Design review of the part built by this model. Coordinates are the model's own, in mm. A direction names the side the tool comes from. Coordinates: 2 decimals unless noted, no trailing zeros. Loops run counter-clockwise (first coordinate to the right, second up) from the corner with the lowest first, then second, coordinate; pieces in that order, holes last. Notation, with made-up numbers: (40.5, -12) -> (71.5, -12) arc R19 ccw to (71.5, 3) -> close; hole circle Ø6 at (30.5, 65). An arc over 180 degrees is marked (long way). One line per item, written item: value. Start each with the question number.
1. Add section A-A on y = 0. Write out the cut boundary in (x, z), plus the area to 3 significant figures.
2. Add section D-D on y = 8. Write out the cut boundary in (x, z).
3. Insertion check: pin 1 (3 mm diameter, centred on x = -20.5, y = -6.5, fed in from +Z); pin 2 (2.5 mm diameter, centred on y = -5, z = 9, fed in from +X); pin 3 (3 mm diameter, centred on x = -3, y = -9, fed in from +Z); pin 4 (2.5 mm diameter, centred on y = -11, z = 4.5, fed in from -X). Each pin has a flat end and moves straight along its axis. Give the tip position at first contact, or say it passes through.
4. Add section C-C on z = 9.5. Write out the cut boundary in (x, y).
5. Draft analysis for pull direction Z (two halves, no side actions). For faces 1 (the flat face through (-13.2, 0.2, 7.8)), 2 (the flat face through (-9, 14.5, 5)), 3 (the flat face through (-14, -4, 4)), 4 (the flat face through (-14, 0, 6.1)), state which applies: pulls with the +Z half, pulls with the -Z half, needs draft (parallel to the pull), parting line crosses it, or undercut.
6. Add section B-B on x = -6.5. Write out the cut boundary in (y, z).
7. For probe 1 along Y at (x, z) = (-8, 4.25); probe 2 along Y at (x, z) = (-14, 10); probe 3 along X at (y, z) = (-11.25, 10), list the stretches that pass through material, from the lowest coordinate up.
8. Machinability: for faces 5 (the flat face through (-4, -10, 4)), 6 (the flat face through (-18, 10, 5)), 7 (the flat face through (-14, 4, 4)), 8 (the flat face through (-15.65, 0, 9)), 9 (the flat face through (-18, -11, 5)), which of the approach directions +Z, -Z, +X, -X, +Y, -Y give a long, thin tool a straight path to every point of the face, cutting with its end or side? Answer none if there is none.
Autodesk Inventor part; units mm, degrees
ref_plane "YZ Plane" through (0, 0, 0) normal (1, 0, 0) x (0, 1, 0)
ref_plane "XZ Plane" through (0, 0, 0) normal (0, 1, 0) x (-1, 0, 0)
ref_plane "XY Plane" through (0, 0, 0) normal (0, 0, 1) x (1, 0, 0)
sketch "Sketch2" plane through (0, 0, 0) normal (0, 0, 1) x (1, 0, 0)
  line L0 (-18, 14.5) -> (18, 14.5)
  line L1 (18, 14.5) -> (18, -14.5)
  line L2 (18, -14.5) -> (-18, -14.5)
  line L3 (-18, -14.5) -> (-18, 14.5)
  line L4 (-18, 14.5) -> (18, -14.5) construction
  line L5 (18, 14.5) -> (-18, -14.5) construction
  point P0 (0, 0)
  dimension "d0" = 29
  dimension "d1" = 36
extrude "Extrusion1" add sketch "Sketch2" along normal blind 11
sketch "Sketch3" plane through (0, 0, 11) normal (0, 0, 1) x (1, 0, 0)
  line L0 (-15.65, 12.15) -> (15.65, 12.15)
  line L1 (15.65, 12.15) -> (15.65, -12.15)
  line L2 (15.65, -12.15) -> (-15.65, -12.15)
  line L3 (-15.65, -12.15) -> (-15.65, 12.15)
  line L4 (-15.65, 12.15) -> (15.65, -12.15) construction
  line L5 (15.65, 12.15) -> (-15.65, -12.15) construction
  point P0 (0, 0)
  dimension "d4" = 31.3
  dimension "d5" = 24.3
extrude "Extrusion2" cut sketch "Sketch3" against normal blind 3.2
sketch "Sketch4" plane through (0, 0, 7.8) normal (0, 0, 1) x (1, 0, 0)
  line L0 (-8, 10) -> (8, 10)
  line L1 (13, 5) -> (13, -6)
  line L2 (9, -10) -> (-9, -10)
  line L3 (-13, -6) -> (-13, 5)
  line L4 (-13, 10) -> (13, -10) construction
  line L5 (13, 10) -> (-13, -10) construction
  line L6 (-13, 5) -> (-8, 10)
  line L7 (8, 10) -> (13, 5)
  arc A0 (-13, -6) -> (-9, -10) centre (-9, -6) ccw
  arc A1 (9, -10) -> (13, -6) centre (9, -6) ccw
  point P0 (0, 0)
  point P1 (-13, -4)
  point P2 (13, -4)
  dimension "d8" = 26
  dimension "d9" = 20
  dimension "d10" = 5
  dimension "d11" = 5
  dimension "d12" = 5
  dimension "d13" = 5
  dimension "d14" = 4
extrude "Extrusion3" cut sketch "Sketch4" against normal through all
sketch "Sketch6" plane through (0, 0, 0) normal (0, 1, 0) x (-1, 0, 0)
  line L0 (13, 7.8) -> (13, 0)
  line L1 (13, 6.1) -> (15.1, 6.1)
  line L2 (15.1, 6.1) -> (13, 1.1)
  line L3 (13, 1.1) -> (13, 6.1)
  line L4 (15.65, 7.8) -> (-15.65, 7.8)
  line L5 (0, 0) -> (0, 10.1915) construction
  line L6 (-13, 7.8) -> (-13, 0)
  line L7 (-13, 6.1) -> (-15.1, 6.1)
  line L8 (-15.1, 6.1) -> (-13, 1.1)
  line L9 (-13, 1.1) -> (-13, 6.1)
  line L10 (-15.65, 7.8) -> (15.65, 7.8)
  dimension "d23" = 2.1
  dimension "d24" = 5
  dimension "d25" = 1.7
extrude "Extrusion5" cut sketch "Sketch6" along normal mid plane 8
sketch "Sketch7" plane through (0, 0, 11) normal (0, 0, 1) x (1, 0, 0)
  arc A0 (21.3831, -3.7533) -> (21.3831, 3.7533) centre (20, 0) ccw
  line L0 (21.3831, 3.7533) -> (18, 5)
  line L1 (18, 5) -> (18, -5)
  line L2 (13, 5) -> (13, -6)
  line L3 (18, -5) -> (21.3831, -3.7533)
  line L4 (0, 20.7674) -> (0, -20.7674) construction
  arc A1 (-21.3831, 3.7533) -> (-21.3831, -3.7533) centre (-20, 0) ccw
  line L5 (-21.3831, 3.7533) -> (-18, 5)
  line L6 (-18, 5) -> (-18, -5)
  line L7 (-18, -5) -> (-21.3831, -3.7533)
  line L8 (18, -14.5) -> (18, 14.5) construction
  circle A2 centre (20, 0) radius 1.65
  circle A3 centre (-20, 0) radius 1.65
  line L9 (0, 0) -> (1.9739, 0) construction
  dimension "d28" = 3.3
  dimension "d29" = 4
  dimension "d30" = 40
  dimension "d31" = 10
extrude "Extrusion6" add sketch "Sketch7" against normal up to surface (11 mm away)
fillet "Fillet1" radius 2 4 edges at (18, -5, 5.5) (18, 5, 5.5) (-18, 5, 5.5) (-18, -5, 5.5)
sketch "Sketch8" plane through (0, 0, 0) normal (1, 0, 0) x (0, 1, 0)
  line L0 (45.1511, -28.2394) -> (-45.1511, -28.2394)
  line L1 (-45.1511, -28.2394) -> (-45.1511, 28.2394)
  line L2 (-45.1511, 28.2394) -> (45.1511, 28.2394)
  line L3 (45.1511, 28.2394) -> (45.1511, -28.2394)
  line L4 (45.1511, -28.2394) -> (-45.1511, 28.2394) construction
  line L5 (-45.1511, -28.2394) -> (45.1511, 28.2394) construction
  point P0 (0, 0)
extrude "Extrusion7" cut sketch "Sketch8" along normal through all
equation "\"d11\" = d10"
equation "\"d12\" = d10"
equation "\"d13\" = d12"
properties part number "power_signal_socket_fixed2" material "Acetal Resin, Black"
Worked answers:
1. outline: (-24, 0) -> (-21.65, 0) -> (-21.65, 11) -> (-24, 11) -> close; (-18.35, 0) -> (-13, 0) -> (-13, 1.1) -> (-15.1, 6.1) -> (-13, 6.1) -> (-13, 7.8) -> (-15.65, 7.8) -> (-15.65, 11) -> (-18.35, 11) -> close
1. area: 71.0 mm²
2. outline: (-18, 0) -> (-10, 0) -> (-10, 7.8) -> (-15.65, 7.8) -> (-15.65, 11) -> (-18, 11) -> close
3. pin 1: passes through
3. pin 2: stops at x = -13
3. pin 3: stops at z = 7.8
3. pin 4: stops at x = -18
4. outline: (-21.38, -3.75) -> (-19.31, -4.52) arc R2 cw to (-18, -6.39) -> (-18, -14.5) -> (0, -14.5) -> (0, -12.15) -> (-15.65, -12.15) -> (-15.65, 12.15) -> (0, 12.15) -> (0, 14.5) -> (-18, 14.5) -> (-18, 6.39) arc R2 cw to (-19.31, 4.52) -> (-21.38, 3.75) arc R4 ccw to start; hole circle Ø3.3 at (-20, 0)
5. face 1: pulls with the +Z half
5. face 2: needs draft
5. face 3: undercut
5. face 4: undercut
6. outline: (-14.5, 0) -> (-10, 0) -> (-10, 7.8) -> (-12.15, 7.8) -> (-12.15, 11) -> (-14.5, 11) -> close; (10, 0) -> (14.5, 0) -> (14.5, 11) -> (12.15, 11) -> (12.15, 7.8) -> (10, 7.8) -> close
7. probe 1: y = -14.5 to -10, 10 to 14.5
7. probe 2: y = -14.5 to -12.15, 12.15 to 14.5
7. probe 3: x = -18 to -15.65
8. face 5: +Z, -Z, +X
8. face 6: +Z, -Z, -X, +Y
8. face 7: +X
8. face 8: +Z, +X
8. face 9: +Z, -Z, -X, -Y
